Check sheet for the modelled part. Datum: model origin and axes. Units: mm. Face numbers are marked on the shaded views. A direction names the side the tool comes from. Give positions to 0.01 mm unless a question says otherwise; leave off trailing zeros. Loops run counter-clockwise (first coordinate to the right, second up) from the corner with the lowest first, then second, coordinate; pieces in that order, holes last.
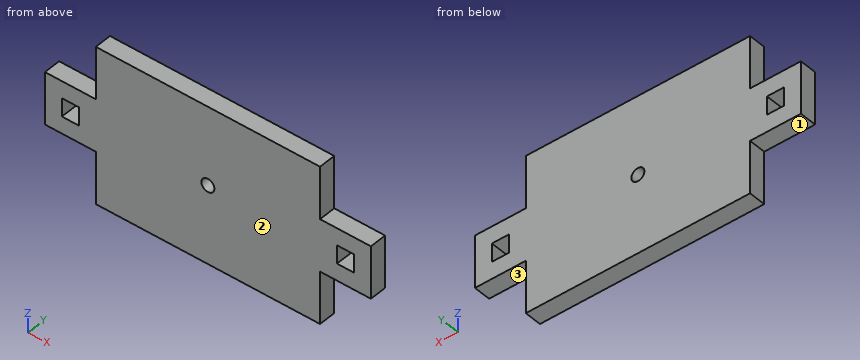
```python
from build123d import *

# Parameters (mm, degrees)
SKETCH1_W           = 125
SKETCH1_H           = 60
BOSS_EXTRUDE1_DEPTH = 6.5
CUT_EXTRUDE1_REACH  = 140.807
SKETCH2_W           = 19.5
SKETCH2_H           = 20
CUT_EXTRUDE2_REACH  = 140.807
SKETCH3_R           = 2.5
CUT_EXTRUDE3_REACH  = 140.807
SKETCH6_W           = 6.5
SKETCH6_H           = 7


with BuildPart() as part:
    # Sketch1 → Boss-Extrude1 (new body)
    with BuildSketch(Plane(origin=(0, 0, 0), x_dir=(1, 0, 0), z_dir=(0, 1, 0))):
        with Locations((62.5, 30)):
            Rectangle(SKETCH1_W, SKETCH1_H)
    extrude(amount=BOSS_EXTRUDE1_DEPTH)

    # Sketch2 → Cut-Extrude1 (cut, up to next)
    with BuildSketch(Plane(origin=(0, 6.5, 0), x_dir=(1, 0, 0), z_dir=(0, 1, 0)), mode=Mode.PRIVATE) as cut_extrude1_sk1:
        with Locations((9.75, 50)):
            Rectangle(SKETCH2_W, SKETCH2_H)
    cut_extrude1_tool1 = extrude(cut_extrude1_sk1.sketch, amount=-CUT_EXTRUDE1_REACH, mode=Mode.PRIVATE) & part.part
    # Sketch2 → Cut-Extrude1 (cut, up to next)
    with BuildSketch(Plane(origin=(0, 6.5, 0), x_dir=(1, 0, 0), z_dir=(0, 1, 0)), mode=Mode.PRIVATE) as cut_extrude1_sk2:
        with Locations((9.75, 10)):
            Rectangle(SKETCH2_W, SKETCH2_H)
    cut_extrude1_tool2 = extrude(cut_extrude1_sk2.sketch, amount=-CUT_EXTRUDE1_REACH, mode=Mode.PRIVATE) & part.part
    # Sketch2 → Cut-Extrude1 (cut, up to next)
    with BuildSketch(Plane(origin=(0, 6.5, 0), x_dir=(1, 0, 0), z_dir=(0, 1, 0)), mode=Mode.PRIVATE) as cut_extrude1_sk3:
        with Locations((115.25, 50)):
            Rectangle(SKETCH2_W, SKETCH2_H)
    cut_extrude1_tool3 = extrude(cut_extrude1_sk3.sketch, amount=-CUT_EXTRUDE1_REACH, mode=Mode.PRIVATE) & part.part
    # Sketch2 → Cut-Extrude1 (cut, up to next)
    with BuildSketch(Plane(origin=(0, 6.5, 0), x_dir=(1, 0, 0), z_dir=(0, 1, 0)), mode=Mode.PRIVATE) as cut_extrude1_sk4:
        with Locations((115.25, 10)):
            Rectangle(SKETCH2_W, SKETCH2_H)
    cut_extrude1_tool4 = extrude(cut_extrude1_sk4.sketch, amount=-CUT_EXTRUDE1_REACH, mode=Mode.PRIVATE) & part.part
    add(cut_extrude1_tool1.solids().sort_by_distance((9.75, 6.5, -50))[0], mode=Mode.SUBTRACT)
    add(cut_extrude1_tool2.solids().sort_by_distance((9.75, 6.5, -10))[0], mode=Mode.SUBTRACT)
    add(cut_extrude1_tool3.solids().sort_by_distance((115.25, 6.5, -50))[0], mode=Mode.SUBTRACT)
    add(cut_extrude1_tool4.solids().sort_by_distance((115.25, 6.5, -10))[0], mode=Mode.SUBTRACT)

    # Sketch3 → Cut-Extrude2 (cut, up to next)
    with BuildSketch(Plane(origin=(0, 6.5, 0), x_dir=(1, 0, 0), z_dir=(0, 1, 0)), mode=Mode.PRIVATE) as cut_extrude2_sk1:
        with Locations(Location((62.5, 30, 0), (0, 0, 270))):
            Circle(SKETCH3_R)
    cut_extrude2_tool1 = extrude(cut_extrude2_sk1.sketch, amount=-CUT_EXTRUDE2_REACH, mode=Mode.PRIVATE) & part.part
    add(cut_extrude2_tool1.solids().sort_by_distance((62.5, 6.5, -30))[0], mode=Mode.SUBTRACT)

    # Sketch6 → Cut-Extrude3 (cut, up to next)
    with BuildSketch(Plane(origin=(0, 6.5, 0), x_dir=(1, 0, 0), z_dir=(0, 1, 0)), mode=Mode.PRIVATE) as cut_extrude3_sk1:
        with Locations((9.75, 30)):
            Rectangle(SKETCH6_W, SKETCH6_H)
    cut_extrude3_tool1 = extrude(cut_extrude3_sk1.sketch, amount=-CUT_EXTRUDE3_REACH, mode=Mode.PRIVATE) & part.part
    # Sketch6 → Cut-Extrude3 (cut, up to next)
    with BuildSketch(Plane(origin=(0, 6.5, 0), x_dir=(1, 0, 0), z_dir=(0, 1, 0)), mode=Mode.PRIVATE) as cut_extrude3_sk2:
        with Locations((115.25, 30)):
            Rectangle(SKETCH6_W, SKETCH6_H)
    cut_extrude3_tool2 = extrude(cut_extrude3_sk2.sketch, amount=-CUT_EXTRUDE3_REACH, mode=Mode.PRIVATE) & part.part
    add(cut_extrude3_tool1.solids().sort_by_distance((9.75, 6.5, -30))[0], mode=Mode.SUBTRACT)
    add(cut_extrude3_tool2.solids().sort_by_distance((115.25, 6.5, -30))[0], mode=Mode.SUBTRACT)


solid = part.part
```
(1) Material ranges on line 1 (X direction, y = 3.25, z = -30); line 2 (X direction, y = 2, z = -2.5); line 3 (Z direction, x = 16, y = 3.75), recorded low to high.
(2) Section check D-D on z = -14.5. Record the boundary of the cut face in (x, y).
(3) Section check C-C on y = 1.25. Record the boundary of the cut face in (x, z), plus the area to 3 significant figures.
(4) Section check A-A on x = 62.5. Record the boundary of the cut face in (y, z), plus the area to 4 significant figures.
(5) Gauge pin test, flat ends, axial feed: pin 1 Ø2 at (x, y) = (10, 3.5) entering from -Z; pin 2 Ø2 at (y, z) = (3, -14) entering from -X; pin 3 Ø3 at (y, z) = (4, -51.5) entering from +X. Record the tip position at first contact, or that the pin passes through.
(6) Section check B-B on z = -30. Record the boundary of the cut face in (x, y).
(7) Access from +Z, -Z, +X, -X, +Y, -Y to the whole of each face (thin tool, end or side, straight path). Record for the marked faces 1, 2 and 3.
Computed values:
1. line 1: x = 0 to 6.5, 13 to 60, 65 to 112, 118.5 to 125
1. line 2: x = 19.5 to 105.5
1. line 3: z = -40 to -20
2. outline: (19.5, 0) - (105.5, 0) - (105.5, 6.5) - (19.5, 6.5) - close
3. outline: (0, -40) - (19.5, -40) - (19.5, -60) - (105.5, -60) - (105.5, -40) - (125, -40) - (125, -20) - (105.5, -20) - (105.5, 0) - (19.5, 0) - (19.5, -20) - (0, -20) - close; hole (6.5, -33.5) - (13, -33.5) - (13, -26.5) - (6.5, -26.5) - close; hole circle Ø5 at (62.5, -30); hole (112, -33.5) - (118.5, -33.5) - (118.5, -26.5) - (112, -26.5) - close
3. area: 5,830 mm2
4. outline: (0, -60) - (6.5, -60) - (6.5, -32.5) - (0, -32.5) - close; (0, -27.5) - (6.5, -27.5) - (6.5, 0) - (0, 0) - close
4. area: 357.5 mm2
5. pin 1: stops at z = -40
5. pin 2: stops at x = 19.5
5. pin 3: stops at x = 105.5
6. outline: (0, 0) - (6.5, 0) - (6.5, 6.5) - (0, 6.5) - close; (13, 0) - (60, 0) - (60, 6.5) - (13, 6.5) - close; (65, 0) - (112, 0) - (112, 6.5) - (65, 6.5) - close; (118.5, 0) - (125, 0) - (125, 6.5) - (118.5, 6.5) - close
7. face 1: -Z, -X, +Y, -Y
7. face 2: +Z, -Z, +X, -X, -Y
7. face 3: -Z, +X, +Y, -Y
